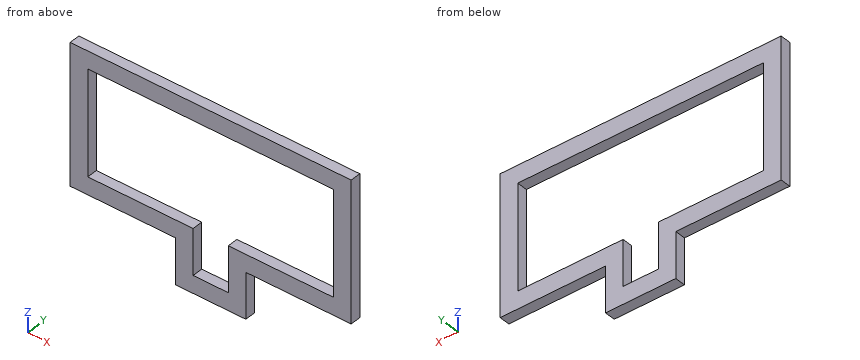
```python
from build123d import *

# Parameters (mm, degrees)
BOSS_EXTRUDE4_DEPTH = 30


with BuildPart() as part:
    # Sketch1 → Boss-Extrude4 (new body)
    with BuildSketch(Plane(origin=(0, 0, 0), x_dir=(1, 0, 0), z_dir=(0, 1, 0))):
        Polygon((-99.811676083, 163.465160075), (-399.811676083, 163.465160075), (-399.811676083, -236.534839925), (400.188323917, -236.534839925), (400.188323917, 163.465160075), (100.188323917, 163.465160075), (50.188323917, 163.465160075), (50.188323917, 113.465160075), (350.188323917, 113.465160075), (350.188323917, -186.534839925), (-349.811676083, -186.534839925), (-349.811676083, 113.465160075), (-49.811676083, 113.465160075), (-49.811676083, 163.465160075), align=None)
        Polygon((-99.811676083, 293.948122897), (-99.811676083, 163.465160075), (-49.811676083, 163.465160075), (-49.811676083, 243.948122897), (50.188323917, 243.948122897), (50.188323917, 163.465160075), (100.188323917, 163.465160075), (100.188323917, 293.948122897), align=None)
    extrude(amount=BOSS_EXTRUDE4_DEPTH)


solid = part.part
```
Geometry check sheet. Reference: the model listing, model coordinates, mm. Give positions to 0.01 mm unless a question says otherwise; leave off trailing zeros. Write each loop counter-clockwise with the first axis right and the second up, starting at its lowest first coordinate (ties: lowest second). Pieces come first, ordered by that corner, then holes.
1) Gauge pin test, flat ends, axial feed: pin 1 (9 mm diameter, centred on x = -279.5, y = 17, fed in from -Z); pin 2 (5 mm diameter, centred on y = 11.5, z = -189.5, fed in from +X). Record the tip position at first contact, or that the pin passes through.
2) Section check C-C, the plane y = 14.5. Record the boundary of the cut face in (x, z).
3) Section check A-A, the plane z = -137.5. Record the boundary of the cut face in (x, y).
4) Material ranges on L1, parallel to X at y = 6.25, z = -149.5; L2, parallel to X at y = 8.25, z = -214; L3, parallel to Z at x = 152, y = 25.25, recorded low to high.
5) Section check B-B, the plane x = 58.5. Record the boundary of the cut face in (y, z).
Computed:
1. pin 1: stops at z = -163.47
1. pin 2: stops at x = 100.19
2. outline: (-399.81, -163.47) - (-99.81, -163.47) - (-99.81, -293.95) - (100.19, -293.95) - (100.19, -163.47) - (400.19, -163.47) - (400.19, 236.53) - (-399.81, 236.53) - close; hole (-349.81, -113.47) - (-49.81, -113.47) - (-49.81, -243.95) - (50.19, -243.95) - (50.19, -113.47) - (350.19, -113.47) - (350.19, 186.53) - (-349.81, 186.53) - close
3. outline: (-399.81, 0) - (-49.81, 0) - (-49.81, 30) - (-399.81, 30) - close; (50.19, 0) - (400.19, 0) - (400.19, 30) - (50.19, 30) - close
4. L1: x = -399.81 to -49.81, 50.19 to 400.19
4. L2: x = -99.81 to -49.81, 50.19 to 100.19
4. L3: z = -163.47 to -113.47, 186.53 to 236.53
5. outline: (0, -293.95) - (30, -293.95) - (30, -113.47) - (0, -113.47) - close; (0, 186.53) - (30, 186.53) - (30, 236.53) - (0, 236.53) - close
